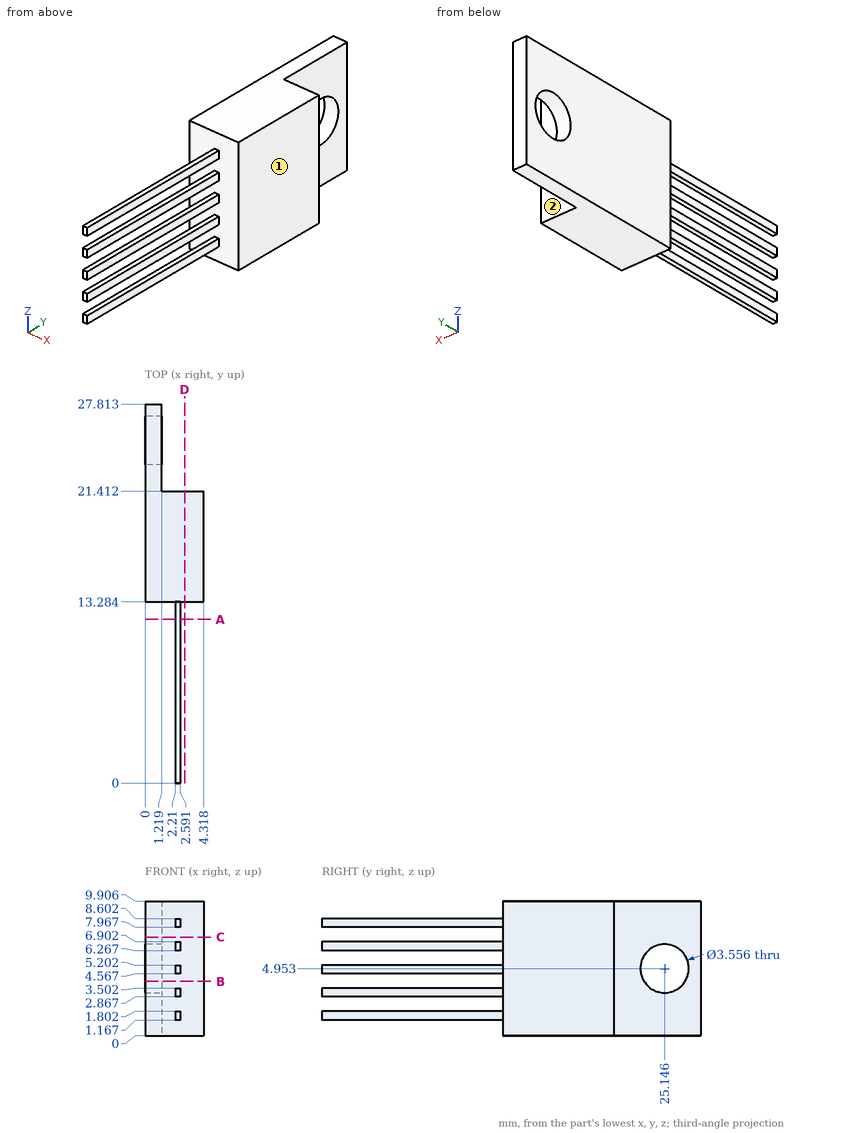
Can you work these out from the drawing? Everything is in mm from the part's minimum corner. A direction names the side the tool comes from. Round coordinates to 2 decimals unless told otherwise and drop trailing zeros. Write each loop counter-clockwise with the first axis right and the second up, starting at its lowest first coordinate (ties: lowest second). Pieces come first, ordered by that corner, then holes. Notation, with made-up numbers: (-8.5, 56) - (36.5, 56) arc R20 cw to (36.5, 76) - close; hole circle Ø1 at (75.5, 39). An arc over 180 degrees is marked (long way). Use a Markdown table: item, result.
Q1. Please list where these lines run through material, in increasing order: L1, parallel to X at y = 26.5, z = 7.5; L2, parallel to Y at x = 2.5, z = 3.25; L3, parallel to X at y = 5.75, z = 8.
Output values:
| item | result |
|---|---|
| L1 | 0 to 1.22 |
| L2 | 0 to 21.41 |
| L3 | 2.21 to 2.59 |
Q2. I want a section at A-A (y = 12). List the corners of the cut face in (x, z) for me.
Output values:
| item | result |
|---|---|
| outline | (2.21, 1.17) - (2.59, 1.17) - (2.59, 1.8) - (2.21, 1.8) - close; (2.21, 2.87) - (2.59, 2.87) - (2.59, 3.5) - (2.21, 3.5) - close; (2.21, 4.57) - (2.59, 4.57) - (2.59, 5.2) - (2.21, 5.2) - close; (2.21, 6.27) - (2.59, 6.27) - (2.59, 6.9) - (2.21, 6.9) - close; (2.21, 7.97) - (2.59, 7.97) - (2.59, 8.6) - (2.21, 8.6) - close |
Q3. For pin 1 (0.7 mm diameter, centred on y = 7, z = 1.5, fed in from -X); pin 2 (0.7 mm diameter, centred on y = 4, z = 3, fed in from +X); pin 3 (2.5 mm diameter, centred on x = 3.5, z = 6, fed in from +Y), each with a flat end and sliding along its axis, tell me the tip position at first contact or that it passes through.
Output values:
| item | result |
|---|---|
| pin 1 | x = 2.21 |
| pin 2 | x = 2.59 |
| pin 3 | y = 21.41 |
Q4. For the marked faces 1 and 2, which set-ups out of +Z, -Z, +X, -X, +Y, -Y let a thin tool reach every point of the face, with its end or its side?
Output values:
| item | result |
|---|---|
| face 1 | +Z, -Z, +X, +Y, -Y |
| face 2 | +Z, -Z, +X, +Y |
Q5. I want a section at C-C (z = 7.25). List the corners of the cut face in (x, y) for me.
Output values:
| item | result |
|---|---|
| outline | (0, 13.28) - (4.32, 13.28) - (4.32, 21.41) - (1.22, 21.41) - (1.22, 27.81) - (0, 27.81) - close |
Q6. I want a section at D-D (x = 2.9). List the corners of the cut face in (y, z) for me, plus the area to 3 significant figures.
Output values:
| item | result |
|---|---|
| outline | (13.28, 0) - (21.41, 0) - (21.41, 9.91) - (13.28, 9.91) - close |
| area | 80.5 mm2 |
Q7. I want a section at B-B (z = 4). List the corners of the cut face in (x, y) for me (1 decimal).
Output values:
| item | result |
|---|---|
| outline | (0, 13.3) - (4.3, 13.3) - (4.3, 21.4) - (1.2, 21.4) - (1.2, 23.6) - (0, 23.6) - close; (0, 26.6) - (1.2, 26.6) - (1.2, 27.8) - (0, 27.8) - close |
